Design review of the part built by this model. Coordinates are the model's own, in mm. A direction names the side the tool comes from. Round coordinates to 2 decimals unless told otherwise and drop trailing zeros. Order: outer loops, then holes, each group sorted by start corner. A loop starts at its lowest first (then second) coordinate and runs counter-clockwise, first axis right, second up.
from build123d import *

# Parameters (mm, degrees)
SKETCH1_W             = 50.8
SKETCH1_H             = 31.75
CUT_EXTRUDE1_DEPTH    = 43.18
CUT_EXTRUDE2_DEPTH    = 43.18
CUT_EXTRUDE3_DEPTH    = 43.18
M36_CLEARANCE_HOLE1_D = 38.1
FILLET1_R             = 5.08
FILLET2_R             = 0.254


with BuildPart() as part:
    # Sketch1 → Revolve1 (revolve)
    with BuildSketch(Plane(origin=(0, 0, 0), x_dir=(-1, 0, 0), z_dir=(0, 0, -1)), mode=Mode.PRIVATE) as revolve1_sk:
        with Locations((-25.4, 15.875)):
            Rectangle(SKETCH1_W, SKETCH1_H)
    revolve(revolve1_sk.sketch.rotate(Axis((50.8, 0, 0), (-1, 0, 0)), 270), axis=Axis((50.8, 0, 0), (-1, 0, 0)))

    # Sketch2 → Cut-Extrude1 (cut)
    with BuildSketch(Plane(origin=(50.8, 0, 0), x_dir=(0, 0, -1), z_dir=(1, 0, 0))):
        with BuildLine():
            ThreePointArc((-17.574990767, 23.012380049), (-25.076631592, 14.478), (-28.716801108, 3.714198451))
            ThreePointArc((-28.716801108, 3.714198451), (-6.467131306, 3.7338), (-17.574990767, 23.012380049))
        make_face()
    extrude(amount=-CUT_EXTRUDE1_DEPTH, mode=Mode.SUBTRACT)

    # Sketch3 → Cut-Extrude2 (cut)
    with BuildSketch(Plane(origin=(50.8, 0, 0), x_dir=(0, 0, -1), z_dir=(1, 0, 0))):
        with BuildLine():
            ThreePointArc((-11.141810341, -26.7265785), (0, -28.956), (11.141810341, -26.7265785))
            ThreePointArc((11.141810341, -26.7265785), (0, -7.4676), (-11.141810341, -26.7265785))
        make_face()
    extrude(amount=-CUT_EXTRUDE2_DEPTH, mode=Mode.SUBTRACT)

    # Sketch4 → Cut-Extrude3 (cut)
    with BuildSketch(Plane(origin=(50.8, 0, 0), x_dir=(0, 0, -1), z_dir=(1, 0, 0))):
        with BuildLine():
            ThreePointArc((28.716801108, 3.714198451), (25.076631592, 14.478), (17.574990767, 23.01238005))
            ThreePointArc((17.574990767, 23.01238005), (6.467131305, 3.7338), (28.716801108, 3.714198451))
        make_face()
    extrude(amount=-CUT_EXTRUDE3_DEPTH, mode=Mode.SUBTRACT)

    # M36 Clearance Hole1 (through all)
    with Locations(Plane.ZY):
        with Locations((0, 0)):
            Hole(M36_CLEARANCE_HOLE1_D / 2)

    # Fillet1
    fillet1_edges = [part.edges().sort_by_distance(p)[0] for p in [
        (29.21, 23.012380049, 17.574990767),
        (29.21, 3.714198451, 28.716801108),
        (29.21, -26.7265785, 11.141810341),
        (29.21, -26.7265785, -11.141810341),
        (29.21, 3.714198451, -28.716801108),
        (29.21, 23.01238005, -17.574990767),
    ]]
    fillet(fillet1_edges, radius=FILLET1_R)

    # Fillet2
    fillet2_edges = [part.edges().sort_by_distance(p)[0] for p in [
        (29.21, 17.654613605, -7.156613617),
        (29.21, -2.629497604, -18.867650684),
        (29.21, 17.654613605, 7.156613618),
        (29.21, -15.025116, -11.711037067),
        (29.21, -15.025116, 11.711037067),
        (29.21, -2.629497604, 18.867650684),
    ]]
    fillet(fillet2_edges, radius=FILLET2_R)


solid = part.part
1) Take a section at B-B on y = -8.5. Give the boundary of the cut face in (x, z).
Results:
outline: (0, -30.59) - (50.8, -30.59) - (50.8, -17.05) - (0, -17.05) - close; (0, 17.05) - (50.8, 17.05) - (50.8, 30.59) - (0, 30.59) - close
2) Take a section at C-C on x = 4.5. Give the boundary of the cut face in (y, z), plus the area to 3 significant figures.
Results:
outline: circle Ø63.5 at (0, 0); hole circle Ø38.1 at (0, 0)
area: 2,030 mm2
3) The part is to be moulded in two halves that separate along Y. For faces 3 (the face through (25.044, -30.995, -6.883)), 4 (the face through (0, -14, -14)), 5 (the face through (29.51, -1.24, 23.53)), say which applies: released by +Y, released by -Y, zero draft, split by the parting line, or undercut.
Results:
face 3: split by the parting line
face 4: zero draft
face 5: undercut
4) For faces 1 (the face through (20.11, -11.59, 15.12)), 2 (the face through (7.62, 10, -20)), list the 3-axis set-ups (+Z, -Z, +X, -X, +Y, -Y) from which the entire face can be reached by the end or side of a thin tool; tool diameter is ignored.
Results:
face 1: +X, -X
face 2: +X
5) Take a section at D-D on y = 10.5. Give the boundary of the cut face in (x, z), plus the area to 3 significant figures.
Results:
outline: (0, -29.96) - (50.8, -29.96) - (50.8, -26.99) - (7.62, -26.99) - (7.62, -15.9) - (0, -15.9) - close; (0, 15.9) - (7.62, 15.9) - (7.62, 26.99) - (50.8, 26.99) - (50.8, 29.96) - (0, 29.96) - close
area: 472 mm2
6) Take a section at A-A on z = 0. Give the boundary of the cut face in (x, y), plus the area to 3 significant figures.
Results:
outline: (0, -31.75) - (50.8, -31.75) - (50.8, -28.96) - (7.62, -28.96) - (7.62, -19.05) - (0, -19.05) - close; (0, 19.05) - (50.8, 19.05) - (50.8, 31.75) - (0, 31.75) - close
area: 863 mm2
7) To check wall thickness, follow line 1 along Y through (x, z) = (37, 0); line 2 along X through (y, z) = (7, -26); line 3 along Y through (x, z) = (4.5, -0.5). State the ranges of each line that lie inside material, in increasing order.
Results:
line 1: y = -31.75 to -28.96, 19.05 to 31.75
line 2: x = 0 to 7.62
line 3: y = -31.75 to -19.04, 19.04 to 31.75
8) Clearance check with flat-ended pins moving along their axes: P1, Ø5, axis at x = 29, z = 8, coming from the -Y side; P2, Ø1.5, axis at x = 39.5, y = 12.5, coming from the +Z side; P3, Ø10, axis at x = 19.5, z = -20, coming from the +Y side. State where each tip first meets the part, or that it passes through.
Results:
P1: stops at y = -31.27
P2: stops at z = 29.5
P3: stops at y = 27.98
